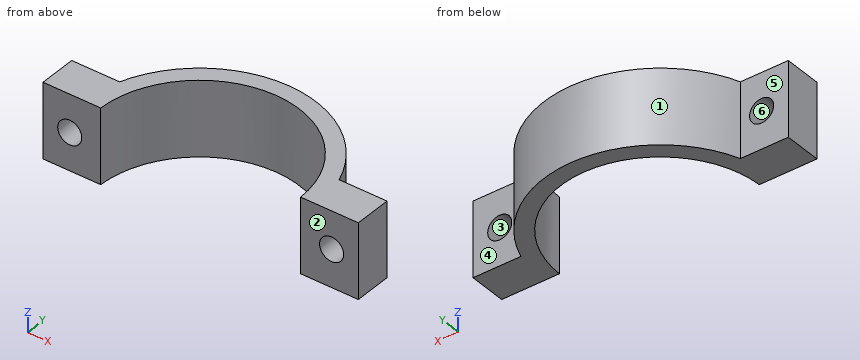
```python
from build123d import *

# Parameters (mm, degrees)
BOLTED_CAP_AND_EARS_DEPTH   = 14
M4_THROUGH_HOLES_DEPTH      = 60.969492244
M4_THROUGH_HOLES_DEPTH_BACK = 60.969492244
SKETCH2_R                   = 2.25


with BuildPart() as part:
    # Bolted cap and ears profile → Bolted cap and ears (new body)
    with BuildSketch(Plane.XY):
        with BuildLine():
            Line((20.541421567, 35.8), (29.5, 35.8))
            Line((29.5, 35.8), (29.5, 28.8))
            Line((29.5, 28.8), (18.697593428, 28.8))
            ThreePointArc((18.697593428, 28.8), (0, 47.2), (-18.697593428, 28.8))
            Line((-18.697593428, 28.8), (-29.5, 28.8))
            Line((-29.5, 28.8), (-29.5, 35.8))
            Line((-29.5, 35.8), (-20.541421567, 35.8))
            ThreePointArc((-20.541421567, 35.8), (0, 50.3), (20.541421567, 35.8))
        make_face()
    extrude(amount=BOLTED_CAP_AND_EARS_DEPTH)

    # Sketch2 → M4 through holes (cut, two sides: drawn at the far end of the back side and taken through both)
    with BuildSketch(Plane(origin=(0, 0, 0), x_dir=(1, 0, 0), z_dir=(0, 1, 0)).offset(-M4_THROUGH_HOLES_DEPTH_BACK)):
        with Locations(Location((-24.5, -7, 0), (0, 0, 90))):
            Circle(SKETCH2_R)
        with Locations(Location((24.5, -7, 0), (0, 0, 90))):
            Circle(SKETCH2_R)
    extrude(amount=M4_THROUGH_HOLES_DEPTH + M4_THROUGH_HOLES_DEPTH_BACK, mode=Mode.SUBTRACT)


solid = part.part
```
Here's how the part is built. I have some questions about the finished solid (model axes, mm). Face numbers are marked on the shaded views. A direction names the side the tool comes from. Coordinates: 2 decimals unless noted, no trailing zeros. Order: outer loops, then holes, each group sorted by start corner. A loop starts at its lowest first (then second) coordinate and runs counter-clockwise, first axis right, second up.
1) Imagine slicing it at C-C on y = 43.75. List the corners of the cut face in (x, z) for me, and give its area (3 significant figures).
2) Will these pins go through, and if not, where does the flat tip stop? pin 1 (2.5 mm diameter, centred on x = -27, z = 9.5, fed in from +Y); pin 2 (2 mm diameter, centred on x = 14, z = 8.5, fed in from -Y); pin 3 (6 mm diameter, centred on y = 44, z = 3.5, fed in from -X).
3) Imagine slicing it at A-A on x = 24.5. List the corners of the cut face in (y, z) for me, and give its area (3 significant figures).
4) We'd pull the mould along X, two halves only. Please class the marked faces 1, 2 and 3: +X half, -X half, draft (parallel to the pull), parting line (faces both ways), or undercut.
5) Which directions (+Z, -Z, +X, -X, +Y, -Y) give clear straight access to the entire face, cutting with the end or side of a thin tool? Please do the marked faces 4, 5 and 6.
6) Imagine slicing it at D-D on y = 35. List the corners of the cut face in (x, z) for me.
7) I need wall thicknesses on line 1 (X direction, y = 30.75, z = 7); line 2 (X direction, y = 33.75, z = 7); line 3 (X direction, y = 42, z = 2.5). Which ranges of each line are inside material? Lowest first, please.
Response values:
1. outline: (-15.58, 0) - (-10.82, 0) - (-10.82, 14) - (-15.58, 14) - close; (10.82, 0) - (15.58, 0) - (15.58, 14) - (10.82, 14) - close
1. area: 133 mm2
2. pin 1: stops at y = 35.8
2. pin 2: stops at y = 39.67
2. pin 3: stops at x = -17.86
3. outline: (28.8, 0) - (35.8, 0) - (35.8, 4.75) - (28.8, 4.75) - close; (28.8, 9.25) - (35.8, 9.25) - (35.8, 14) - (28.8, 14) - close
3. area: 66.5 mm2
4. face 1: parting line
4. face 2: draft
4. face 3: undercut
5. face 4: +Z, -Z, +X, +Y
5. face 5: +Z, -Z, -X, +Y
5. face 6: +Y, -Y
6. outline: (-29.5, 0) - (-17.53, 0) - (-17.53, 14) - (-29.5, 14) - close; (17.53, 0) - (29.5, 0) - (29.5, 14) - (17.53, 14) - close; hole circle Ø4.5 at (-24.5, 7); hole circle Ø4.5 at (24.5, 7)
7. line 1: x = -29.5 to -26.75, -22.25 to -18.56, 18.56 to 22.25, 26.75 to 29.5
7. line 2: x = -29.5 to -26.75, -22.25 to -17.95, 17.95 to 22.25, 26.75 to 29.5
7. line 3: x = -17.12 to -12.94, 12.94 to 17.12
